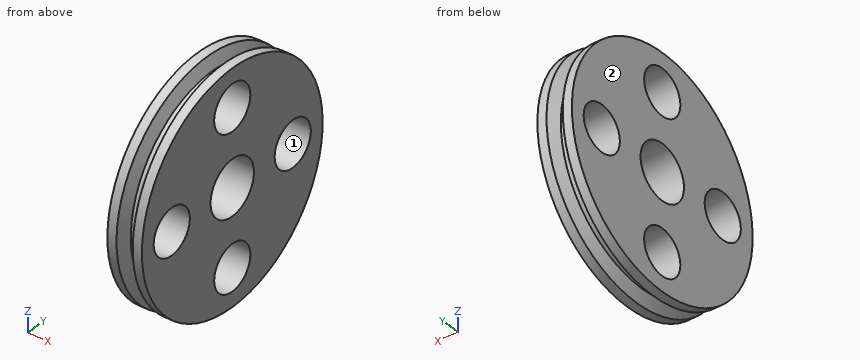
from build123d import *

# Parameters (mm, degrees)
SKETCH2_R          = 20
CUT_EXTRUDE1_DEPTH = 103
CIRPATTERN1_COUNT  = 4


with BuildPart() as part:
    # Sketch1 → Revolve1 (revolve)
    with BuildSketch(Plane.XY, mode=Mode.PRIVATE) as revolve1_sk:
        Polygon((-20.854858804, 24), (-51.021525471, 24), (-51.021525471, 100), (-43.021525471, 100), (-38.438192137, 90), (-33.438192137, 90), (-28.854858804, 100), (-20.854858804, 100), align=None)
    revolve(revolve1_sk.sketch.rotate(Axis((0, 0, 0), (-1, 0, 0)), 90), axis=Axis((0, 0, 0), (-1, 0, 0)))

    # Sketch2 → Cut-Extrude1 (cut)
    with BuildSketch(Plane(origin=(-20.854858804, 0, 0), x_dir=(0, 0, -1), z_dir=(1, 0, 0))):
        with Locations((0, 66.936858639)):
            Circle(SKETCH2_R)
    cut_extrude1 = extrude(amount=-CUT_EXTRUDE1_DEPTH, mode=Mode.SUBTRACT)

    # CirPattern1: Cut-Extrude1 ×4 about axis
    cirpattern1_axis = Axis((0, 0, 0), (1, 0, 0))
    for i in range(1, CIRPATTERN1_COUNT):
        add(cut_extrude1.rotate(cirpattern1_axis, i * 360 / CIRPATTERN1_COUNT), mode=Mode.SUBTRACT)


solid = part.part
Work out the finished part from the listing and answer in its coordinate system (mm). Face numbers are marked on the shaded views. Give positions to 0.01 mm unless a question says otherwise; leave off trailing zeros. Loops run counter-clockwise (first coordinate to the right, second up) from the corner with the lowest first, then second, coordinate; pieces in that order, holes last. Notation, with made-up numbers: (43, 58.5) - (70, 58.5) arc R26 ccw to (70, 75.5) - close; hole circle Ø8 at (-16.75, -1). An arc over 180 degrees is marked (long way). Answer in a Markdown table with one row per item. Add a question column.
Q1. Consider line 1 along Y through (x, z) = (-37, 0); line 2 along Z through (x, y) = (-37, -2); line 3 along Y through (x, z) = (-40.5, 4). Determine where each line is inside the solid, lowest interval first.
Q2. Each of these flat-tipped pins is pushed along its axis until it touches: P1, Ø1.5, axis at x = -27, y = 45.5, coming from the -Z side; P2, Ø6, axis at x = -33, z = -0.5, coming from the +Y side; P3, Ø1, axis at x = -34.5, z = 9, coming from the -Y side. Where does it stop, or does it pass through?
Q3. The part is cut by section A-A (z = 0). Determine the outline of the cut face in (x, y).
Q4. Determine the mould class of the marked faces 1 and 2 for opening direction Y: released by +Y, released by -Y, zero draft, split by the parting line, or undercut.
Solution:
| question | item | result |
|---|---|---|
| 1 | line 1 | y = -90 to -86.94, -46.94 to -24, 24 to 46.94, 86.94 to 90 |
| 1 | line 2 | z = -89.98 to -86.84, -47.04 to -23.92, 23.92 to 47.04, 86.84 to 89.98 |
| 1 | line 3 | y = -94.41 to -86.53, -47.34 to -23.66, 23.66 to 47.34, 86.53 to 94.41 |
| 2 | P1 | stops at z = -89.43 |
| 2 | P2 | stops at y = 97.5 |
| 2 | P3 | stops at y = -89.6 |
| 3 | outline | (-51.02, -100) - (-43.02, -100) - (-38.44, -90) - (-33.44, -90) - (-28.85, -100) - (-20.85, -100) - (-20.85, -86.94) - (-51.02, -86.94) - close; (-51.02, -46.94) - (-20.85, -46.94) - (-20.85, -24) - (-51.02, -24) - close; (-51.02, 24) - (-20.85, 24) - (-20.85, 46.94) - (-51.02, 46.94) - close; (-51.02, 86.94) - (-20.85, 86.94) - (-20.85, 100) - (-28.85, 100) - (-33.44, 90) - (-38.44, 90) - (-43.02, 100) - (-51.02, 100) - close |
| 4 | face 1 | undercut |
| 4 | face 2 | zero draft |
